```python
from build123d import *

# Parameters (mm, degrees)
F0_W     = 457.2
F0_H     = 304.8
F1_DEPTH = 44.45
F3_DEPTH = 457.201
F5_DEPTH = 44.451
F7_DEPTH = 304.801


with BuildPart() as f1:
    # F0 (on Front) → F1 (new body)
    with BuildSketch(Plane.XZ):
        with Locations((154.513133, 152.4)):
            Rectangle(F0_W, F0_H)
    extrude(amount=F1_DEPTH)

    # F2 (on face) → F3 (cut, through all)
    with BuildSketch(Plane.YZ.offset(383.113133)):
        Polygon((-44.45, 101.6), (-12.7, 304.8), (-82.839599, 304.8), (-82.839599, 0), (-12.7, 0), align=None)
    extrude(amount=-F3_DEPTH, mode=Mode.SUBTRACT)

    # F4 (on face) → F5 (cut, through all)
    with BuildSketch(Plane(origin=(0, 0, 0), x_dir=(-1, 0, 0), z_dir=(0, 1, 0))):
        Polygon((74.086867, 304.8), (-332.313133, 304.8), (74.086867, 101.6), align=None)
    extrude(amount=-F5_DEPTH, mode=Mode.SUBTRACT)

    # F6 (on face) → F7 (cut, through all)
    with BuildSketch(Plane(origin=(0, 0, 0), x_dir=(1, 0, 0), z_dir=(0, 0, -1))):
        Polygon((332.313133, 0), (383.113133, 0), (383.113133, 50.8), align=None)
    extrude(amount=-F7_DEPTH, mode=Mode.SUBTRACT)


solid = f1.part
```
The listing builds one solid part. Answer for the finished solid, in the listing's coordinates (mm). Round coordinates to 2 decimals unless told otherwise and drop trailing zeros. Order: outer loops, then holes, each group sorted by start corner. A loop starts at its lowest first (then second) coordinate and runs counter-clockwise, first axis right, second up. Notation, with made-up numbers: (72, 87.5) - (85, 87.5) arc R12 cw to (85, 93.5) - close; hole circle Ø5 at (64.5, 64.25). An arc over 180 degrees is marked (long way). Put each result on its own line as item: value. Start each with the question number.
(1) Find section C-C (z = 63). Give the vertices of the cut face in (x, y).
(2) Find section A-A (x = 200.5). Give the vertices of the cut face in (y, z).
(3) Straight lines are drawn through the part: probe 1 along Y at (x, z) = (246.5, 125); probe 2 along X at (y, z) = (-25.5, 220); probe 3 along Y at (x, z) = (-8, 40). For each, find the intervals that lie inside material, in ascending order. Write a range as from..to.
(4) Given P1, Ø1, axis at x = 285, z = 191.5, coming from the -Y side; P2, Ø1.5, axis at x = 133, z = 121, coming from the +Y side; P3, Ø3, axis at x = 133, z = 42.5, coming from the -Y side; P4, Ø5, axis at y = -5.5, z = 236, coming from the -X side, each flat-ended and moving along its own axis, determine where each tip first touches the part or whether it passes through.
(5) Find section B-B (y = -35). Give the vertices of the cut face in (x, z).
(6) Find section D-D (z = 223). Give the vertices of the cut face in (x, y).
Reply:
1. outline: (-74.09, -32.39) - (364.7, -32.39) - (332.31, 0) - (-74.09, 0) - close
2. outline: (-44.45, 101.6) - (-12.7, 0) - (0, 0) - (0, 238.89) - (-23, 238.89) - close
3. probe 1: -40.79..0
3. probe 2: 162.71..357.81
3. probe 3: -25.2..0
4. P1: y = -30.48
4. P2: y = 0
4. P3: y = -26.45
4. P4: x = 189.71
5. outline: (-74.09, 71.36) - (367.31, 71.36) - (367.31, 162.08) - (46.87, 162.08) - (-74.09, 101.6) - close
6. outline: (168.71, -25.48) - (357.79, -25.48) - (332.31, 0) - (168.71, 0) - close
